Autodesk Inventor part; units mm, degrees
ref_plane "YZ Plane" through (0, 0, 0) normal (1, 0, 0) x (0, 1, 0)
ref_plane "XZ Plane" through (0, 0, 0) normal (0, 1, 0) x (-1, 0, 0)
ref_plane "XY Plane" through (0, 0, 0) normal (0, 0, 1) x (1, 0, 0)
sketch "Эскиз1" plane through (0, 0, 0) normal (0, 0, 1) x (1, 0, 0)
  line L0 (0, 0) -> (1, 0)
  line L1 (10, 0) -> (10, -3)
  line L2 (10, -3) -> (3, -3)
  line L3 (0, -3) -> (0, 0)
  line L4 (0, -3) -> (-7.3989, -3)
  line L5 (-7.3989, -3) -> (-7.3989, -5) construction
  line L6 (-7.3989, -5) -> (0, -5)
  line L7 (0, -5) -> (0, -3) construction
  line L8 (0, -3) -> (2, -3) construction
  line L9 (2, -4) -> (2, -4)
  line L10 (1, -5) -> (0, -5)
  line L11 (0, -5) -> (0, -3) construction
  line L12 (-7.3989, -3) -> (-6, 0)
  line L13 (-7.3989, -3) -> (-13.5, -3) construction
  line L14 (-57.3989, -3) -> (-57.3989, -5) construction
  line L15 (-57.3989, -5) -> (-7.3989, -5)
  line L16 (-7.3989, -5) -> (-7.3989, -3) construction
  arc A0 (1, -5) -> (2, -4) centre (1, -4) ccw
  arc A1 (3, -3) -> (2, -4) centre (3, -4) ccw
  line L17 (-13.5, -3) -> (-17.5, -3) construction
  line L18 (0, 0) -> (1, 0)
  line L19 (10, 0) -> (9, 0)
  arc A2 (1, 0) -> (9, 0) centre (5, 9.1652) ccw
  line L20 (-57.3989, -3) -> (-60.6335, -3)
  line L21 (-60.6335, -3) -> (-62.2492, -12.1633)
  line L22 (-62.2492, -12.8686) -> (-58.2492, -12.8686) construction
  line L23 (-58.2492, -12.8686) -> (-58.2492, -9.8223) construction
  line L24 (-58.2492, -12.8686) -> (6.2271, -24.2375)
  line L25 (6.2271, -24.2375) -> (6.7481, -21.2831)
  line L26 (6.7481, -21.2831) -> (-58.2492, -9.8223)
  line L27 (-58.2492, -9.8223) -> (-58.2492, -12.8686) construction
  line L28 (-57.3989, -5) -> (-57.3989, -3) construction
  line L29 (-58.2492, -9.8223) -> (-57.3989, -5)
  line L30 (-13.5, -3) -> (-17.5, -3) construction
  line L31 (-17.5, -3) -> (-57.3989, -3)
  line L32 (1, 0) -> (9, 0) construction
  line L33 (9, 0) -> (10, 0)
  line L34 (-58.2492, -12.8686) -> (-62.2492, -12.1633)
  line L35 (-62.2492, -12.1633) -> (-62.2492, -12.8686) construction
  line L36 (-6, 0) -> (-7.5, 0) construction
  line L37 (-7.5, 0) -> (-7.5, -3) construction
  line L38 (-7.5, 0) -> (-9.5, 0) construction
  line L39 (-7.5, 0) -> (-9.5, 0) construction
  line L40 (-9.5, 0) -> (-13.5, -3) construction
  line L41 (-13.5, -3) -> (-17.5, -3) construction
  spline S0 degree 3 poles (-7.5, 0) (-9.5, 0) (-13.5, -3) (-17.5, -3) knots 1 1 1 1 2 2 2 2
  line L42 (-7.5, 0) -> (-6, 0)
  point P0 (2, -5)
  point P1 (0, -5)
  dimension "d0" = 10
  dimension "d1" = 3
  dimension "d3" = 2
  dimension "d4" = 2
  dimension "d5" = 2
  dimension "d6" = 50
  dimension "d9" = 1
  dimension "d10" = 1
  dimension "d11" = 4
  dimension "d13" = 2
  dimension "d14" = 1
  dimension "d15" = 1
  dimension "d16" = 10
  dimension "d17" = 4
  dimension "d18" = 10
  dimension "d20" = 3
  dimension "d21" = 65.471
  dimension "d25" = 4.8967
  dimension "d26" = 66
  dimension "d27" = 90
  dimension "d28" = 100
  dimension "d29" = 65
  dimension "d30" = 6
  dimension "d31" = 3
  dimension "d32" = 1.5
  dimension "d33" = 6
  dimension "d34" = 2
extrude "Выдавливание1" add sketch "Эскиз1" along normal blind 15
properties part number "bat_lock01"
Source: CAD feature listing. Evaluate the final solid. Frame: model axes, mm. A direction names the side the tool comes from. Give positions to 0.01 mm unless a question says otherwise; leave off trailing zeros. Loops run counter-clockwise (first coordinate to the right, second up) from the corner with the lowest first, then second, coordinate; pieces in that order, holes last. Notation, with made-up numbers: (18.5, 80) -> (23.5, 80) arc R7 cw to (23.5, 87) -> close; hole circle Ø2 at (-4, 20). An arc over 180 degrees is marked (long way). Use a Markdown table: item, result. Add a question column.
1) Line query: line 1 along Y through (x, z) = (-6.5, 6.5); line 2 along Y through (x, z) = (-30.5, 5.75); line 3 along Y through (x, z) = (-39.5, 12). Output: solid intervals per line, ascending. Write a range as [from, to].
2) Pull-direction query (X, two-part tool) for faces 1 (the face through (-28, -5, 7)), 2 (the face through (-6.7, -1.5, 7.4)), 3 (the face through (-57.83, -7.44, 7.4)); classes: +X half, -X half, draft (parallel to the pull), parting line (faces both ways), or undercut.
3) Reachability of faces 4 (the face through (0, -2, 7)), 5 (the face through (-39, -3, 7)), 6 (the face through (-4, -3, 7)), 7 (the face through (-7, 0, 7)), 8 (the face through (-25.296, -15.633, 7.395)) from +Z, -Z, +X, -X, +Y, -Y: full face, straight path, thin tool, end or side. Return the list, or none.
4) Section query A-A, the plane x = -34. Return the cut outline in (y, z), then the cut area to 3 significant figures.
5) Section query B-B, the plane y = -16.25. Return the cut outline in (x, z), then the cut area to 3 significant figures.
6) Section query C-C, the plane y = -8.75. Return the cut outline in (x, z), then the cut area to 3 significant figures.
7) First-contact query: pin 1 (5 mm diameter, centred on y = -7, z = 10.5, fed in from -X); pin 2 (1 mm diameter, centred on x = -55, z = 2, fed in from +Y); pin 3 (2 mm diameter, centred on x = -13.5, z = 11, fed in from -Y). Flat tips, straight axial feed; report the tip coordinate or a pass-through.
Numbers:
| question | item | result |
|---|---|---|
| 1 | line 1 | y = [-21.99, -18.95], [-5, -3], [-1.07, 0] |
| 1 | line 2 | y = [-17.76, -14.72], [-5, -3] |
| 1 | line 3 | y = [-16.17, -13.13], [-5, -3] |
| 2 | face 1 | draft |
| 2 | face 2 | undercut |
| 2 | face 3 | +X half |
| 3 | face 4 | +Z, -Z, +Y |
| 3 | face 5 | +Z, -Z, -X, +Y |
| 3 | face 6 | +Z, -Z |
| 3 | face 7 | +Z, -Z, +X, -X, +Y |
| 3 | face 8 | +Z, -Z, +X |
| 4 | outline | (-17.14, 0) -> (-14.1, 0) -> (-14.1, 15) -> (-17.14, 15) -> close; (-5, 0) -> (-3, 0) -> (-3, 15) -> (-5, 15) -> close |
| 4 | area | 75.7 mm2 |
| 5 | outline | (-39.07, 0) -> (-21.8, 0) -> (-21.8, 15) -> (-39.07, 15) -> close |
| 5 | area | 259 mm2 |
| 6 | outline | (-61.65, 0) -> (-58.06, 0) -> (-58.06, 15) -> (-61.65, 15) -> close |
| 6 | area | 53.8 mm2 |
| 7 | pin 1 | stops at x = -61.78 |
| 7 | pin 2 | stops at y = -3 |
| 7 | pin 3 | stops at y = -20.94 |
